Check sheet for the drawn part. Datum: minimum x, y, z corner. Units: mm. Give positions to 0.01 mm unless a question says otherwise; leave off trailing zeros. Order: outer loops, then holes, each group sorted by start corner. A loop starts at its lowest first (then second) coordinate and runs counter-clockwise, first axis right, second up. Notation, with made-up numbers: M 89,64.5 L 126,64.5 A10 ccw 126,73.5 Z; hole C -22,69 d9. An arc over 180 degrees is marked long. One line per question, with ' | ' between items. Start each with the question number.
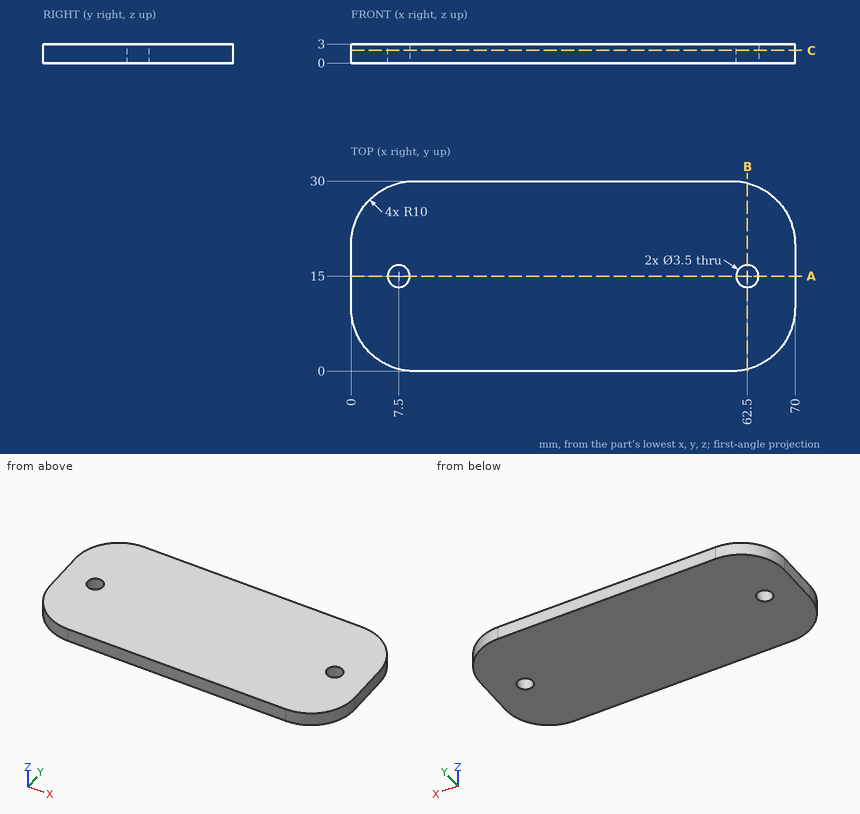
Item 1: Section check C-C, the plane z = 2. Record the cut outline in (x, y), then the cut area to 3 significant figures.
Item 2: Go/stop test with flat-tipped pins: P1, Ø1.5, axis at y = 4, z = 2, coming from the -X side; P2, Ø1, axis at y = 23.5, z = 0.5, coming from the +X side. Record where each tip stops, or that it passes through.
Item 3: Section check B-B, the plane x = 62.5. Record the cut outline in (y, z).
Item 4: Scan lines: probe 1 along Y at (x, z) = (62.5, 1.3); probe 2 along Y at (x, z) = (8, 0.6); probe 3 along X at (y, z) = (24.5, 1). Record each from-to range of solid material in increasing order. Write a range as [from, to].
Item 5: Section check A-A, the plane y = 15. Record the cut outline in (x, z), then the cut area to 3 significant figures.
Reported:
1) outline: M 0,10 A10 ccw 10,0 L 60,0 A10 ccw 70,10 L 70,20 A10 ccw 60,30 L 10,30 A10 ccw 0,20 Z; hole C 7.5,15 d3.5; hole C 62.5,15 d3.5 | area: 1,990 mm^2
2) P1: stops at x = 1.49 | P2: stops at x = 69.54
3) outline: M 0.32,0 L 13.25,0 L 13.25,3 L 0.32,3 Z; M 16.75,0 L 29.68,0 L 29.68,3 L 16.75,3 Z
4) probe 1: y = [0.32, 13.25], [16.75, 29.68] | probe 2: y = [0.2, 13.32], [16.68, 29.8] | probe 3: x = [1.07, 68.93]
5) outline: M 0,0 L 5.75,0 L 5.75,3 L 0,3 Z; M 9.25,0 L 60.75,0 L 60.75,3 L 9.25,3 Z; M 64.25,0 L 70,0 L 70,3 L 64.25,3 Z | area: 189 mm^2
